```python
from build123d import *

# Parameters (mm, degrees)
ESQUISSE1_W             = 20
ESQUISSE1_H             = 13
BOSS_EXTRU_1_DEPTH      = 20
ESQUISSE2_R             = 3
ENL_V_MAT_EXTRU_1_DEPTH = 20
ESQUISSE3_R             = 1.5
ENL_V_MAT_EXTRU_2_DEPTH = 20
CONG_1_R                = 1
CONG_2_R                = 0.5
CONG_3_R                = 0.5
CONG_4_R                = 0.5
CONG_5_R                = 0.5
CONG_6_R                = 1
ESQUISSE4_R             = 9
ESQUISSE4_R_2           = 3
ENL_V_MAT_EXTRU_3_DEPTH = 0.5


with BuildPart() as part:
    # Esquisse1 → Boss.-Extru.1 (new body)
    with BuildSketch(Plane(origin=(0, 0, 0), x_dir=(1, 0, 0), z_dir=(0, 1, 0))):
        Rectangle(ESQUISSE1_W, ESQUISSE1_H)
    extrude(amount=BOSS_EXTRU_1_DEPTH)

    # Esquisse2 → Enlèv. mat.-Extru.1 (cut)
    with BuildSketch(Plane.XY.offset(6.5)):
        with Locations((0, 10)):
            Circle(ESQUISSE2_R)
    extrude(amount=-ENL_V_MAT_EXTRU_1_DEPTH, mode=Mode.SUBTRACT)

    # Esquisse3 → Enlèv. mat.-Extru.2 (cut)
    with BuildSketch(Plane(origin=(0, 20, 0), x_dir=(1, 0, 0), z_dir=(0, 1, 0))):
        with Locations((-7, 2)):
            Circle(ESQUISSE3_R)
        with Locations((7, 2)):
            Circle(ESQUISSE3_R)
    extrude(amount=-ENL_V_MAT_EXTRU_2_DEPTH, mode=Mode.SUBTRACT)

    # Congé1
    cong_1_edges = [part.edges().sort_by_distance(p)[0] for p in [
        (-3, 10, 6.5),
    ]]
    fillet(cong_1_edges, radius=CONG_1_R)

    # Congé2
    cong_2_edges = [part.edges().sort_by_distance(p)[0] for p in [
        (-8.5, 20, -2),
    ]]
    fillet(cong_2_edges, radius=CONG_2_R)

    # Congé3
    cong_3_edges = [part.edges().sort_by_distance(p)[0] for p in [
        (5.5, 20, -2),
    ]]
    fillet(cong_3_edges, radius=CONG_3_R)

    # Congé4
    cong_4_edges = [part.edges().sort_by_distance(p)[0] for p in [
        (-8.5, 0, -2),
    ]]
    fillet(cong_4_edges, radius=CONG_4_R)

    # Congé5
    cong_5_edges = [part.edges().sort_by_distance(p)[0] for p in [
        (5.5, 0, -2),
    ]]
    fillet(cong_5_edges, radius=CONG_5_R)

    # Congé6
    cong_6_edges = [part.edges().sort_by_distance(p)[0] for p in [
        (-3, 10, -6.5),
    ]]
    fillet(cong_6_edges, radius=CONG_6_R)

    # Esquisse4 → Enlèv. mat.-Extru.3 (cut)
    with BuildSketch(Plane.XY.offset(6.5)):
        with Locations((0, 10)):
            Circle(ESQUISSE4_R)
        with Locations((0, 10)):
            Circle(ESQUISSE4_R_2, mode=Mode.SUBTRACT)
    enl_v_mat_extru_3 = extrude(amount=-ENL_V_MAT_EXTRU_3_DEPTH, mode=Mode.SUBTRACT)

    # Symétrie1: Enlèv. mat.-Extru.3 across plane
    add(enl_v_mat_extru_3.mirror(Plane.XY), mode=Mode.SUBTRACT)


solid = part.part
```
Could you check a few things on this model? Use its own coordinates, in mm. A direction names the side the tool comes from. Coordinates: 2 decimals unless noted, no trailing zeros. Loops run counter-clockwise (first coordinate to the right, second up) from the corner with the lowest first, then second, coordinate; pieces in that order, holes last.
1) Please list where these lines run through material, in increasing order: line 1 along Z through (x, y) = (7, 7.5); line 2 along X through (y, z) = (18, -3.25); line 3 along Y through (x, z) = (0, -6.15).
Reported:
line 1: z = -6 to -3.5, -0.5 to 6
line 2: x = -10 to -7.83, -6.17 to 6.17, 7.83 to 10
line 3: y = 0 to 1, 19 to 20
2) Imagine slicing it at A-A (y = 10). List the corners of the cut face in (x, z) for me, and give its area (3 significant figures).
Reported:
outline: (-10, -6.5) - (-9, -6.5) - (-9, -6) - (-3.13, -6) arc R1 ccw to (-3, -5.5) - (-3, 5.5) arc R1 ccw to (-3.13, 6) - (-9, 6) - (-9, 6.5) - (-10, 6.5) - close; (3, -5.5) arc R1 ccw to (3.13, -6) - (9, -6) - (9, -6.5) - (10, -6.5) - (10, 6.5) - (9, 6.5) - (9, 6) - (3.13, 6) arc R1 ccw to (3, 5.5) - close; hole circle Ø3 at (-7, -2); hole circle Ø3 at (7, -2)
area: 156 mm2
3) Will this pin go through, and if not, where does the flat tip stop? pin 1 Ø9 at (x, y) = (-1, 11.5) entering from +Z.
Reported:
pin 1: stops at z = 6
4) Thinking about a two-plate mould opening in X: for faces 1 (the face through (0, 6, 6)), 2 (the face through (-10, 10, 0)), 3 (the face through (-2, 1, -6.5)), which applies, released by +X, released by -X, zero draft, split by the parting line, or undercut?
Reported:
face 1: undercut
face 2: released by -X
face 3: zero draft
5) Which directions (+Z, -Z, +X, -X, +Y, -Y) give clear straight access to the entire face, cutting with the end or side of a thin tool? Please do faces 4 (the face through (-1.951, 1.214, 6.254)), 5 (the face through (-2, 1, 6.5)), 6 (the face through (0, 6, -6)).
Reported:
face 4: +Z
face 5: +Z, +X, -X, +Y, -Y
face 6: -Z
6) Imagine slicing it at C-C (z = -2). List the corners of the cut face in (x, y) for me, and give its area (3 significant figures).
Reported:
outline: (-10, 0) - (-9, 0) arc R0.5 ccw to (-8.5, 0.5) - (-8.5, 19.5) arc R0.5 ccw to (-9, 20) - (-10, 20) - close; (-5.5, 0.5) arc R0.5 ccw to (-5, 0) - (5, 0) arc R0.5 ccw to (5.5, 0.5) - (5.5, 19.5) arc R0.5 ccw to (5, 20) - (-5, 20) arc R0.5 ccw to (-5.5, 19.5) - close; (8.5, 0.5) arc R0.5 ccw to (9, 0) - (10, 0) - (10, 20) - (9, 20) arc R0.5 ccw to (8.5, 19.5) - close; hole circle Ø6 at (0, 10)
area: 251 mm2
7) Imagine slicing it at D-D (y = 4.5). List the corners of the cut face in (x, z) for me.
Reported:
outline: (-10, -6.5) - (-7.12, -6.5) - (-7.12, -6) - (7.12, -6) - (7.12, -6.5) - (10, -6.5) - (10, 6.5) - (7.12, 6.5) - (7.12, 6) - (-7.12, 6) - (-7.12, 6.5) - (-10, 6.5) - close; hole circle Ø3 at (-7, -2); hole circle Ø3 at (7, -2)
8) Imagine slicing it at B-B (x = 0). List the corners of the cut face in (y, z) for me.
Reported:
outline: (0, -6.5) - (1, -6.5) - (1, -6) - (6.87, -6) arc R1 ccw to (7, -5.5) - (7, 5.5) arc R1 ccw to (6.87, 6) - (1, 6) - (1, 6.5) - (0, 6.5) - close; (13, -5.5) arc R1 ccw to (13.13, -6) - (19, -6) - (19, -6.5) - (20, -6.5) - (20, 6.5) - (19, 6.5) - (19, 6) - (13.13, 6) arc R1 ccw to (13, 5.5) - close
